Geometry: final body of the model. Coordinates: model frame, mm. Coordinates: 2 decimals unless noted, no trailing zeros. Order: outer loops, then holes, each group sorted by start corner. A loop starts at its lowest first (then second) coordinate and runs counter-clockwise, first axis right, second up. Notation, with made-up numbers: M 58,-14 L 93,-14 A9 ccw 93,3 Z; hole C -0.5,81.5 d4. An arc over 180 degrees is marked long. Write item = value, one per line.
from build123d import *

# Parameters (mm, degrees)
F4_DEPTH = 25


# Not quite as in the source:
# - a feature of the source that left no trace in its solid (it failed there, or was rolled back) is left out
# - the program builds the solid bodies; features that only make, move or delete a surface that nothing else refers to are left out


with BuildPart() as f4:
    # F3 (on face) → F4 (new body)
    with BuildSketch(Plane.YZ.offset(100)):
        Polygon((17.3205080757, 10), (0, 20), (-17.3205080757, 10), (-17.3205080757, -10), (0, -20), (17.3205080757, -10), align=None)
    extrude(amount=F4_DEPTH)


solid = f4.part
1) Section C-C, the plane y = 10. Return loops of the section in (x, z).
Numbers:
outline = M 100,-14.23 L 125,-14.23 L 125,14.23 L 100,14.23 Z
2) Section B-B, the plane z = -12.5. Return loops of the section in (x, y).
Numbers:
outline = M 100,-12.99 L 125,-12.99 L 125,12.99 L 100,12.99 Z
3) Pin query (flat end, axial travel): pin 1 (1 mm diameter, centred on x = 118.5, y = -12.5, fed in from +Z); pin 2 (6 mm diameter, centred on x = 118, y = -10.5, fed in from -Z); pin 3 (5 mm diameter, centred on x = 111, y = 0.5, fed in from -Z). Return the tip coordinate at first contact, or that it passes through.
Numbers:
pin_1 = 13.07
pin_2 = -15.67
pin_3 = -20
4) Section A-A, the plane x = 120.75. Return loops of the section in (y, z).
Numbers:
outline = M -17.32,-10 L 0,-20 L 17.32,-10 L 17.32,10 L 0,20 L -17.32,10 Z
5) Line query: L1, parallel to Y at x = 121.75, z = -13; L2, parallel to Y at x = 110, z = 15; L3, parallel to Z at x = 117.5, y = 6. Output: solid intervals per line, ascending.
Numbers:
L1 = -12.12 to 12.12
L2 = -8.66 to 8.66
L3 = -16.54 to 16.54
